Geometry check sheet. Reference: the model listing, model coordinates, mm. Face numbers are marked on the shaded views. Coordinates: 2 decimals unless noted, no trailing zeros. Order: outer loops, then holes, each group sorted by start corner. A loop starts at its lowest first (then second) coordinate and runs counter-clockwise, first axis right, second up. Notation, with made-up numbers: M 5.5,0 L 17.5,0 A22 cw 17.5,35 Z; hole C 21,25 d11. An arc over 180 degrees is marked long. One line per item, written item: value. Start each with the question number.
1) Sectioned sample at A-A, the plane y = -25. Enter the section's corners in (x, z).
2) Draft check along X on the marked faces 1, 2 and 3. Enter one of: pulls with the +X half, pulls with the -X half, needs draft (parallel to the pull), parting line crosses it, or undercut.
3) Sectioned sample at D-D, the plane z = 15. Enter the section's corners in (x, y).
4) Go/stop test with flat-tipped pins: P1, Ø23, axis at y = -24.6, z = -75.89, coming from the -X side; P2, Ø2, axis at x = -19.5, y = -38.5, coming from the -Z side. Record where each tip stops, or that it passes through.
5) Thickness scan on L1, parallel to Z at x = 31.5, y = -27.5; L2, parallel to X at y = -24, z = 18.5; L3, parallel to Z at x = -48.5, y = -24.6. Record the ranges inside material, lowest first. Write a range as from..to.
6) Sectioned sample at B-B, the plane x = 63. Enter the section's corners in (y, z), then the cut area to 3 significant figures.
7) Sectioned sample at C-C, the plane y = -40. Enter the section's corners in (x, z), then the cut area to 3 significant figures.
```python
from build123d import *

# Parameters (mm, degrees)
F1_DEPTH = 50
F2_R     = 19.05
F3_DEPTH = 25
F4_R     = 19.05
F5_DEPTH = 25


with BuildPart() as f1:
    # F0 (on Front) → F1 (new body)
    with BuildSketch(Plane.XZ):
        with BuildLine():
            Line((-53.070944, 22.410468), (-53.070944, -101.289532))
            Line((-53.070944, -101.289532), (-47.070944, -101.289532))
            Line((-47.070944, -101.289532), (-47.070944, 22.410468))
            ThreePointArc((-47.070944, 22.410468), (-44.142012, 29.481535), (-37.070944, 32.410468))
            Line((-37.070944, 32.410468), (86.629056, 32.410468))
            Line((86.629056, 32.410468), (86.629056, 38.410468))
            Line((86.629056, 38.410468), (-37.070944, 38.410468))
            ThreePointArc((-37.070944, 38.410468), (-48.384652, 33.724176), (-53.070944, 22.410468))
        make_face()
    extrude(amount=F1_DEPTH)

    # F2 (on face) → F3 (cut)
    with BuildSketch(Plane.XY.offset(38.410468)):
        with Locations((56.629056, -25)):
            Circle(F2_R)
    extrude(amount=-F3_DEPTH, mode=Mode.SUBTRACT)

    # F4 (on face) → F5 (cut)
    with BuildSketch(Plane(origin=(-53.070944, 0, 0), x_dir=(0, -1, 0), z_dir=(-1, 0, 0))):
        with Locations((24.6, -75.889532)):
            Circle(F4_R)
    extrude(amount=-F5_DEPTH, mode=Mode.SUBTRACT)


solid = f1.part
```
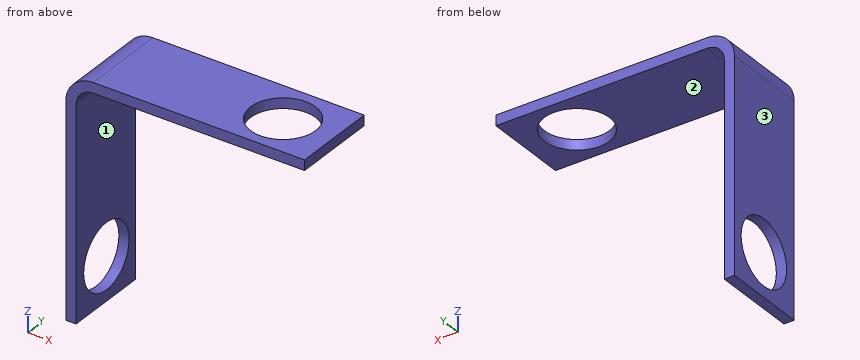
Final values:
1. outline: M -53.07,-101.29 L -47.07,-101.29 L -47.07,-94.94 L -53.07,-94.94 Z; M -53.07,-56.84 L -47.07,-56.84 L -47.07,22.41 A10 cw -37.07,32.41 L 37.58,32.41 L 37.58,38.41 L -37.07,38.41 A16 ccw -53.07,22.41 Z; M 75.68,32.41 L 86.63,32.41 L 86.63,38.41 L 75.68,38.41 Z
2. face 1: pulls with the +X half
2. face 2: needs draft
2. face 3: pulls with the -X half
3. outline: M -53.07,-50 L -47.07,-50 L -47.07,0 L -53.07,0 Z
4. P1: passes through
4. P2: stops at z = 32.41
5. L1: z = 32.41..38.41
5. L2: x = -53.07..-47.07
5. L3: z = -101.29..-94.94, -56.84..33.61
6. outline: M -50,32.41 L -42.95,32.41 L -42.95,38.41 L -50,38.41 Z; M -7.05,32.41 L 0,32.41 L 0,38.41 L -7.05,38.41 Z
6. area: 84.6 mm^2
7. outline: M -53.07,-101.29 L -47.07,-101.29 L -47.07,-87.1 L -53.07,-87.1 Z; M -53.07,-64.68 L -47.07,-64.68 L -47.07,22.41 A10 cw -37.07,32.41 L 44.89,32.41 L 44.89,38.41 L -37.07,38.41 A16 ccw -53.07,22.41 Z; M 68.37,32.41 L 86.63,32.41 L 86.63,38.41 L 68.37,38.41 Z
7. area: 1,330 mm^2
